Input: part model. Units: mm. Frame: model coordinates. Round coordinates to 2 decimals unless told otherwise and drop trailing zeros. Loops run counter-clockwise (first coordinate to the right, second up) from the corner with the lowest first, then second, coordinate; pieces in that order, holes last. Notation, with made-up numbers: (4.5, 88.5) -> (34.5, 88.5) arc R4 ccw to (34.5, 93.5) -> close; hole circle Ø6 at (18, 38). An arc over 180 degrees is marked (long way). Answer in a Markdown table with one row per item. Add a question column.
Q1. Section C-C, the plane x = -0.5. Output: boundary loops of the cut face in (y, z) (3 decimals).
Q2. Pin query (flat end, axial travel): pin 1 (4 mm diameter, centred on y = 0, z = 44.45, fed in from +X). Return the tip coordinate at first contact, or that it passes through.
Q3. Section A-A, the plane z = 0. Output: boundary loops of the cut face in (x, y) (3 decimals), and give its area (3 significant figures).
Q4. Ray query, L1, parallel to Y at x = 1, z = 44.45 (3 decimals); L2, parallel to Z at x = 1.5, y = 1.5; L3, parallel to Y at x = -1.5, z = -2 (3 decimals). Return the intervals inside material, ascending. Write a range as from..to.
Q5. Section B-B, the plane y = 0. Output: boundary loops of the cut face in (x, z) (3 decimals).
Q6. Mould query, pull axis Y, two halves, no side actions, for faces 1 (the face through (-0.04, -2.44, -0.54)), 2 (the face through (0, 9.525, 1)), 3 (the face through (-3.175, 4, 1)). Classes: pulls with the +Y half, pulls with the -Y half, needs draft (parallel to the pull), parting line crosses it, or undercut.
```python
from build123d import *

# Parameters (mm, degrees)
SKETCH1_W                 = 6.35
SKETCH1_H                 = 19.05
EXTRUDE1_DEPTH            = 57.15
M6X1_0_TAPPED_HOLE1_D     = 5
M6X1_0_TAPPED_HOLE1_DEPTH = 6.35
M6X1_0_TAPPED_HOLE2_D     = 5


with BuildPart() as part:
    # Sketch1 → Extrude1 (new body, symmetric)
    with BuildSketch(Plane.XY):
        Rectangle(SKETCH1_W, SKETCH1_H)
    extrude(amount=EXTRUDE1_DEPTH, both=True)

    # M6x1.0 Tapped Hole1
    with Locations(Plane(origin=(3.175, 0, 0), x_dir=(0, 0, -1), z_dir=(1, 0, 0))):
        with Locations((-44.45, 0), (44.45, 0)):
            Hole(M6X1_0_TAPPED_HOLE1_D / 2, depth=M6X1_0_TAPPED_HOLE1_DEPTH)

    # M6x1.0 Tapped Hole2 (through all)
    with Locations(Plane(origin=(3.175, 0, 0), x_dir=(0, 0, -1), z_dir=(1, 0, 0))):
        with Locations((0, 0)):
            Hole(M6X1_0_TAPPED_HOLE2_D / 2)


solid = part.part
```
Answer block:
| question | item | result |
|---|---|---|
| 1 | outline | (-9.525, -57.15) -> (9.525, -57.15) -> (9.525, 57.15) -> (-9.525, 57.15) -> close; hole circle Ø5 at (0, -44.45); hole circle Ø5 at (0, 0); hole circle Ø5 at (0, 44.45) |
| 2 | pin 1 | through |
| 3 | outline | (-3.175, -9.525) -> (3.175, -9.525) -> (3.175, -2.5) -> (-3.175, -2.5) -> close; (-3.175, 2.5) -> (3.175, 2.5) -> (3.175, 9.525) -> (-3.175, 9.525) -> close |
| 3 | area | 89.2 mm^2 |
| 4 | L1 | -9.525..-2.5, 2.5..9.525 |
| 4 | L2 | -57.15..-46.45, -42.45..-2, 2..42.45, 46.45..57.15 |
| 4 | L3 | -9.525..-1.5, 1.5..9.525 |
| 5 | outline | (-3.175, -57.15) -> (3.175, -57.15) -> (3.175, -46.95) -> (-3.175, -46.95) -> close; (-3.175, -41.95) -> (3.175, -41.95) -> (3.175, -2.5) -> (-3.175, -2.5) -> close; (-3.175, 2.5) -> (3.175, 2.5) -> (3.175, 41.95) -> (-3.175, 41.95) -> close; (-3.175, 46.95) -> (3.175, 46.95) -> (3.175, 57.15) -> (-3.175, 57.15) -> close |
| 6 | face 1 | undercut |
| 6 | face 2 | pulls with the +Y half |
| 6 | face 3 | needs draft |
